from build123d import *

# Parameters (mm, degrees)
KES_EKSTR_ZYON1_DEPTH = 431
KES_EKSTR_ZYON2_DEPTH = 24


with BuildPart() as part:
    # Çizim1 → Döndür1 (revolve)
    with BuildSketch(Plane.XY):
        Polygon((-303.5, 0), (303.5, 0), (303.5, 15), (177.5, 15), (177.5, 17.5), (-253.5, 17.5), (-253.5, 15), (-303.5, 15), align=None)
    revolve(axis=Axis((-303.5, 0, 0), (1, 0, 0)))

    # Çizim2 → Kes-Ekstrüzyon1 (cut)
    with BuildSketch(Plane.ZY.offset(253.5)):
        with BuildLine():
            Line((-15, 9.013878189), (-15, -9.013878189))
            ThreePointArc((-15, -9.013878189), (-17.5, 0), (-15, 9.013878189))
        make_face()
        with BuildLine():
            Line((15, 9.013878189), (15, -9.013878189))
            ThreePointArc((15, -9.013878189), (17.5, 0), (15, 9.013878189))
        make_face()
    extrude(amount=-KES_EKSTR_ZYON1_DEPTH, mode=Mode.SUBTRACT)

    # Çizim3 → Kes-Ekstrüzyon2 (cut)
    with BuildSketch(Plane(origin=(0, 0, 0), x_dir=(1, 0, 0), z_dir=(0, 1, 0))):
        with BuildLine():
            Line((297.5, -4), (237.5, -4))
            ThreePointArc((237.5, -4), (233.5, 0), (237.5, 4))
            Line((237.5, 4), (297.5, 4))
            ThreePointArc((297.5, 4), (301.5, 0), (297.5, -4))
        make_face()
    extrude(amount=-KES_EKSTR_ZYON2_DEPTH, mode=Mode.SUBTRACT)


solid = part.part
Verification items for the finished model (mm, model axes). A direction names the side the tool comes from. Round coordinates to 2 decimals unless told otherwise and drop trailing zeros. Write each loop counter-clockwise with the first axis right and the second up, starting at its lowest first coordinate (ties: lowest second). Pieces come first, ordered by that corner, then holes.
(1) Section check A-A (x = 213.5). Enter the section's corners in (y, z).
Returned:
outline: circle Ø30 at (0, 0)
(2) Section check B-B (x = 44). Enter the section's corners in (y, z).
Returned:
outline: (-9.01, -15) - (9.01, -15) arc R17.5 ccw to (9.01, 15) - (-9.01, 15) arc R17.5 ccw to start
(3) Mould release check, pull along Z, two halves, no side actions. Record for faces 5 (the flat face through (267, -7, -4)), 6 (the flat face through (268, -7, 4)), 7 (the cylindrical face through (-41.02, 17.5, -0.25)), 8 (the flat face through (177.5, 15.3, 1.2)): pulls with the +Z half, pulls with the -Z half, needs draft (parallel to the pull), parting line crosses it, or undercut.
Returned:
face 5: undercut
face 6: undercut
face 7: parting line crosses it
face 8: needs draft
(4) Access from +Z, -Z, +X, -X, +Y, -Y to the whole of each face (thin tool, end or side, straight path). Record for faces 1 (the flat face through (-253.5, 15.2, 0.1)), 2 (the cylindrical face through (-278.85, -14.985, 0.66)), 3 (the flat face through (-253.5, -15.3, 1.2)), 4 (the cylindrical face through (239.618, 13.856, -5.745)).
Returned:
face 1: -X, +Y
face 2: -X
face 3: -X, -Y
face 4: +X
(5) Material ranges on line 1 (Z direction, x = 251, y = -12); line 2 (X direction, y = -5.5, z = -1); line 3 (Y direction, x = -140, z = 0), recorded low to high.
Returned:
line 1: z = -9 to -4, 4 to 9
line 2: x = -303.5 to 233.63, 301.37 to 303.5
line 3: y = -17.5 to 17.5
(6) Depth check by flat-ended pin: pin 1 Ø4 at (x, y) = (-164, -13.5) entering from +Z; pin 2 Ø4 at (x, z) = (256, -0.5) entering from -Y; pin 3 Ø8 at (x, z) = (137.5, -10) entering from +Y; pin 4 Ø11.5 at (x, y) = (266, -5) entering from +Z. Enter the tip coordinate at first touch or a pass-through.
Returned:
pin 1: stops at z = 13.19
pin 2: stops at y = 0
pin 3: stops at y = 16.44
pin 4: stops at z = 15
